Input: part model. Units: mm. Frame: model coordinates. Face numbers are marked on the shaded views. A direction names the side the tool comes from. Round coordinates to 2 decimals unless told otherwise and drop trailing zeros. Order: outer loops, then holes, each group sorted by start corner. A loop starts at its lowest first (then second) coordinate and runs counter-clockwise, first axis right, second up. Notation, with made-up numbers: M -15,56.5 L 10,56.5 A34 cw 10,89.5 Z; hole C 2,-29 d7. An arc over 180 degrees is marked long. One line per question, with ' | ' between items.
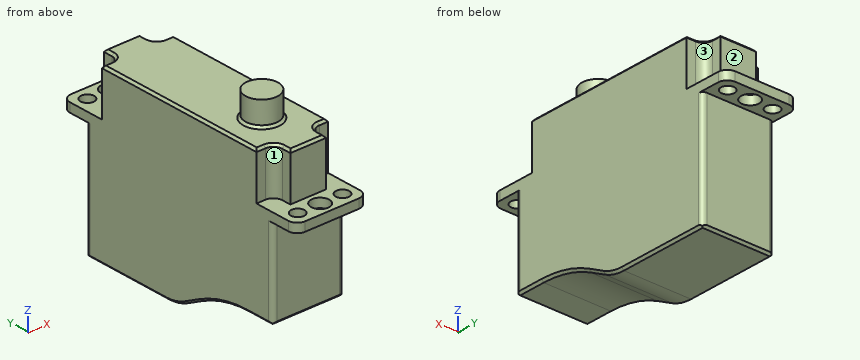
```python
from build123d import *

# Parameters (mm, degrees)
BOSS_EXTRUDE1_DEPTH = 8
SKETCH2_R           = 1
SKETCH2_R_2         = 0.75
CUT_EXTRUDE1_DEPTH  = 31.952746243
FILLET1_R           = 1
SKETCH3_R           = 1.8
BOSS_EXTRUDE2_DEPTH = 2.7
CUT_EXTRUDE2_DEPTH  = 5.15
CHAMFER1_SIZE       = 0.254
CHAMFER2_SIZE       = 0.254
FILLET2_R           = 0.508


with BuildPart() as part:
    # Sketch1 → Boss-Extrude1 (new body)
    with BuildSketch(Plane.YZ):
        with BuildLine():
            Line((0, 0), (23.5, 0))
            Line((23.5, 0), (23.5, -5.15))
            Line((23.5, -5.15), (26.5, -5.15))
            Line((26.5, -5.15), (26.5, -6.15))
            Line((26.5, -6.15), (23.5, -6.15))
            Line((23.5, -6.15), (23.5, -19))
            Line((23.5, -19), (13.321336499, -19))
            ThreePointArc((13.321336499, -19), (12.106318726, -18.852558343), (10.961830178, -18.418792051))
            Line((10.961830178, -18.418792051), (9.120424555, -17.453019871))
            ThreePointArc((9.120424555, -17.453019871), (6.259203186, -16.368604142), (3.221658753, -16))
            Line((3.221658753, -16), (0, -16))
            Line((0, -16), (0, -6.15))
            Line((0, -6.15), (-3, -6.15))
            Line((-3, -6.15), (-3, -5.15))
            Line((-3, -5.15), (0, -5.15))
            Line((0, -5.15), (0, 0))
        make_face()
    extrude(amount=BOSS_EXTRUDE1_DEPTH)

    # Sketch2 → Cut-Extrude1 (cut, through all)
    with BuildSketch(Plane.XY.offset(-5.15)):
        with Locations((4, -1.5)):
            Circle(SKETCH2_R)
        with Locations((4, 25)):
            Circle(SKETCH2_R)
        with Locations((6.5, 25)):
            Circle(SKETCH2_R_2)
        with Locations((1.5, 25)):
            Circle(SKETCH2_R_2)
        with Locations((1.5, -1.5)):
            Circle(SKETCH2_R_2)
        with Locations((6.5, -1.5)):
            Circle(SKETCH2_R_2)
    extrude(amount=-CUT_EXTRUDE1_DEPTH, mode=Mode.SUBTRACT)

    # Fillet1
    fillet1_edges = [part.edges().sort_by_distance(p)[0] for p in [
        (8, -3, -5.65),
        (0, 26.5, -5.65),
        (0, -3, -5.65),
        (8, 26.5, -5.65),
    ]]
    fillet(fillet1_edges, radius=FILLET1_R)

    # Sketch3 → Boss-Extrude2 (add)
    with BuildSketch(Plane.XY):
        with Locations(Location((4, 5.85, 0), (0, 0, 180))):
            Circle(SKETCH3_R)
    extrude(amount=BOSS_EXTRUDE2_DEPTH)

    # Sketch4 → Cut-Extrude2 (cut)
    with BuildSketch(Plane.XY):
        with BuildLine():
            Line((0, 23.5), (2, 23.5))
            Line((2, 23.5), (2, 22.5))
            ThreePointArc((2, 22.5), (1.707106781, 21.792893219), (1, 21.5))
            Line((1, 21.5), (0, 21.5))
            Line((0, 21.5), (0, 23.5))
        make_face()
        with BuildLine():
            Line((8, 23.5), (6, 23.5))
            Line((6, 23.5), (6, 22.5))
            ThreePointArc((6, 22.5), (6.292893219, 21.792893219), (7, 21.5))
            Line((7, 21.5), (8, 21.5))
            Line((8, 21.5), (8, 23.5))
        make_face()
        with BuildLine():
            Line((0, 0), (2, 0))
            Line((2, 0), (2, 1))
            ThreePointArc((2, 1), (1.707106781, 1.707106781), (1, 2))
            Line((1, 2), (0, 2))
            Line((0, 2), (0, 0))
        make_face()
        with BuildLine():
            Line((8, 0), (6, 0))
            Line((6, 0), (6, 1))
            ThreePointArc((6, 1), (6.292893219, 1.707106781), (7, 2))
            Line((7, 2), (8, 2))
            Line((8, 2), (8, 0))
        make_face()
    extrude(amount=-CUT_EXTRUDE2_DEPTH, mode=Mode.SUBTRACT)

    # Chamfer1
    chamfer1_edges = [part.edges().sort_by_distance(p)[0] for p in [
        (5.8, 5.85, 0),
        (0, 11.75, 0),
        (8, 11.75, 0),
        (4, 0, 0),
        (4, 23.5, 0),
        (6, 23, 0),
        (6.292893219, 21.792893219, 0),
        (7.5, 21.5, 0),
        (2, 0.5, 0),
        (1.707106781, 1.707106781, 0),
        (0.5, 2, 0),
        (7.5, 2, 0),
        (6.292893219, 1.707106781, 0),
        (6, 0.5, 0),
        (0.5, 21.5, 0),
        (1.707106781, 21.792893219, 0),
        (2, 23, 0),
    ]]
    chamfer(chamfer1_edges, length=CHAMFER1_SIZE)

    # Chamfer2
    chamfer2_edges = [part.edges().sort_by_distance(p)[0] for p in [
        (0, 18.410668249, -19),
        (0, 12.106318726, -18.852558343),
        (0, 10.041127366, -17.935905961),
        (0, 6.259203186, -16.368604142),
        (0, 1.610829376, -16),
        (8, 1.610829376, -16),
        (4, 23.5, -19),
        (4, 0, -16),
        (8, 6.259203186, -16.368604142),
        (8, 10.041127366, -17.935905961),
        (8, 12.106318726, -18.852558343),
        (8, 18.410668249, -19),
    ]]
    chamfer(chamfer2_edges, length=CHAMFER2_SIZE)

    # Fillet2
    fillet2_edges = [part.edges().sort_by_distance(p)[0] for p in [
        (0, 0, -10.948),
        (8, 0, -10.948),
        (0, 23.5, -12.448),
        (8, 23.5, -12.448),
    ]]
    fillet(fillet2_edges, radius=FILLET2_R)


solid = part.part
```
Item 1: First-contact query: pin 1 (1.1 mm diameter, centred on x = 0.5, z = -2, fed in from -Y); pin 2 (0.8 mm diameter, centred on y = 23, z = -3, fed in from +X); pin 3 (2 mm diameter, centred on x = 1.5, y = 4.5, fed in from -Z). Flat tips, straight axial feed; report the tip coordinate or a pass-through.
Report:
pin 1: y = 2 | pin 2: x = 6 | pin 3: z = -16.21
Item 2: Access query for the marked faces 1, 2 and 3. Directions: +Z, -Z, +X, -X, +Y, -Y. A direction counts if a zero-diameter tool reaches every point of the face in a straight line with its end or side. Return the directions, or none.
Report:
face 1: +Z, -X, -Y | face 2: +Z, +X, -X, +Y | face 3: +Z, +X, +Y
Item 3: Section query B-B, the plane y = 14. Return loops of the section in (x, z), plus the area to 3 significant figures.
Report:
outline: M 0,-18.75 L 0.25,-19 L 7.75,-19 L 8,-18.75 L 8,-0.25 L 7.75,0 L 0.25,0 L 0,-0.25 Z | area: 152 mm²
Item 4: Section query C-C, the plane z = -2.5. Return loops of the section in (x, y), plus the area to 3 significant figures.
Report:
outline: M 0,2 L 1,2 A1 cw 2,1 L 2,0 L 6,0 L 6,1 A1 cw 7,2 L 8,2 L 8,21.5 L 7,21.5 A1 cw 6,22.5 L 6,23.5 L 2,23.5 L 2,22.5 A1 cw 1,21.5 L 0,21.5 Z | area: 173 mm²
Item 5: Section query A-A, the plane y = -1.5. Return loops of the section in (x, z).
Report:
outline: M 0,-6.15 L 0.75,-6.15 L 0.75,-5.15 L 0,-5.15 Z; M 2.25,-6.15 L 3,-6.15 L 3,-5.15 L 2.25,-5.15 Z; M 5,-6.15 L 5.75,-6.15 L 5.75,-5.15 L 5,-5.15 Z; M 7.25,-6.15 L 8,-6.15 L 8,-5.15 L 7.25,-5.15 Z
Item 6: Line query: line 1 along Y through (x, z) = (6.5, -5.45); line 2 along X through (y, z) = (22.5, -3.75); line 3 along Z through (x, y) = (5.75, 15.5). Output: solid intervals per line, ascending. Write a range as from..to.
Report:
line 1: -3..-2.25, -0.75..24.25, 25.75..26.5 | line 2: 2..6 | line 3: -19..0
Item 7: Section query D-D, the plane x = 1.5. Give the number of separate pieces and of enclosed holes in the cut face, plus the area to 3 significant figures.
Report:
separate pieces: 3 | enclosed holes: 0 | area: 403 mm²
